Source: CAD feature listing. Evaluate the final solid. Frame: model axes, mm. A direction names the side the tool comes from. Round coordinates to 2 decimals unless told otherwise and drop trailing zeros. Write each loop counter-clockwise with the first axis right and the second up, starting at its lowest first coordinate (ties: lowest second). Pieces come first, ordered by that corner, then holes. Notation, with made-up numbers: M -12,27.5 L 19,27.5 A9 cw 19,35.5 Z; hole C 30.5,0 d3. An arc over 180 degrees is marked long. Answer in a Markdown table with one row per item. Add a question column.
Item 1: Material intervals for probe 1 along Y at (x, z) = (-14.5, 2.85); probe 2 along X at (y, z) = (-22, 0.7); probe 3 along X at (y, z) = (-40, 2.85), sorted ascending.
Item 2: Cut plane C-C on x = 8. Return loops of the section in (y, z), and give its area (3 significant figures).
Item 3: Set-up query: faces 5 (the face through (0, -24, 0)), 6 (the face through (14.222, -27.236, 1.578)). Return all of +Z, -Z, +X, -X, +Y, -Y with unobstructed straight access to the full face (end or side cutting, diameter ignored); none if empty.
Item 4: Mould query, pull axis X, two halves, no side actions, for faces 1 (the face through (0.58, -57.188, 2.465)), 2 (the face through (3, -42, 3.2)), 3 (the face through (11.753, -23.369, 4.087)), 4 (the face through (-15.837, -36.846, 2.465)). Classes: released by +X, released by -X, zero draft, split by the parting line, or undercut.
Item 5: Cut plane D-D on y = -32. Return loops of the section in (x, z).
Item 6: Cut plane B-B on y = -23. Return loops of the section in (x, z).
Item 7: Cut plane A-A on z = 2.3. Return loops of the section in (x, y).
Item 8: Contact query for flat-ended pins moving along their axis: pin 1 (4 mm diameter, centred on x = 12.5, y = -22.5, fed in from +Z); pin 2 (2 mm diameter, centred on x = -12, y = -24, fed in from -Z); pin 3 (2 mm diameter, centred on y = -43, z = 3.5, fed in from -X); pin 4 (5.5 mm diameter, centred on x = -12.29, y = -24.01, fed in from -Z). Output: stop coordinate, or through.
from build123d import *

# Parameters (mm, degrees)
F0_R     = 4
F0_R_2   = 3.25
F0_R_3   = 2.145
F1_DEPTH = 5
F2_DEPTH = 3.2


with BuildPart() as f1:
    # F0 (on Top) → F1 (new body)
    with BuildSketch(Plane.XY):
        with BuildLine():
            ThreePointArc((-10.6575777754, -53.0245751143), (-5.3198116886, -56.1150509582), (0.7539304934, -57.1885702394))
            ThreePointArc((0.7539304934, -57.1885702394), (6.8276726753, -56.1150509582), (12.1654387622, -53.0245751143))
            ThreePointArc((12.1654387622, -53.0245751143), (17.232310235, -37.0535716462), (27.7539304934, -24.013569904))
            ThreePointArc((27.7539304934, -24.013569904), (0.7539304934, -3.2972529395), (-26.2460695066, -24.013569904))
            ThreePointArc((-26.2460695066, -24.013569904), (-15.7244492482, -37.0535716462), (-10.6575777754, -53.0245751143))
        make_face()
        with BuildLine():
            ThreePointArc((4.7539304934, -41.1667175744), (3.5823576181, -43.9951446991), (0.7539304934, -45.1667175744))
            ThreePointArc((0.7539304934, -45.1667175744), (-3.2460695066, -41.1667175744), (0.7539304934, -37.1667175744))
            ThreePointArc((0.7539304934, -37.1667175744), (3.5823576181, -38.3382904496), (4.7539304934, -41.1667175744))
        make_face(mode=Mode.SUBTRACT)
        with Locations((-12.2910695066, -24.013569904)):
            Circle(F0_R, mode=Mode.SUBTRACT)
        with BuildLine():
            ThreePointArc((17.7989304934, -24.013569904), (13.7989304934, -28.013569904), (9.7989304934, -24.013569904))
            ThreePointArc((9.7989304934, -24.013569904), (13.7989304934, -20.013569904), (17.7989304934, -24.013569904))
        make_face(mode=Mode.SUBTRACT)
        with BuildLine():
            ThreePointArc((17.7989304934, -24.013569904), (13.7989304934, -20.013569904), (9.7989304934, -24.013569904))
            ThreePointArc((9.7989304934, -24.013569904), (13.7989304934, -28.013569904), (17.7989304934, -24.013569904))
        make_face()
        with BuildLine():
            ThreePointArc((17.0489304934, -24.013569904), (13.7989304934, -27.263569904), (10.5489304934, -24.013569904))
            ThreePointArc((10.5489304934, -24.013569904), (13.7989304934, -20.763569904), (17.0489304934, -24.013569904))
        make_face(mode=Mode.SUBTRACT)
        with Locations((-12.2910695066, -24.013569904)):
            Circle(F0_R)
        with Locations((-12.2910695066, -24.013569904)):
            Circle(F0_R_2, mode=Mode.SUBTRACT)
        with BuildLine():
            ThreePointArc((17.0489304934, -24.013569904), (13.7989304934, -20.763569904), (10.5489304934, -24.013569904))
            ThreePointArc((10.5489304934, -24.013569904), (13.7989304934, -27.263569904), (17.0489304934, -24.013569904))
        make_face()
        with BuildLine():
            ThreePointArc((15.9439304934, -24.013569904), (13.7989304934, -26.158569904), (11.6539304934, -24.013569904))
            ThreePointArc((11.6539304934, -24.013569904), (13.7989304934, -21.868569904), (15.9439304934, -24.013569904))
        make_face(mode=Mode.SUBTRACT)
        with Locations((-12.2910695066, -24.013569904)):
            Circle(F0_R_2)
        with Locations((-12.2910695066, -24.013569904)):
            Circle(F0_R_3, mode=Mode.SUBTRACT)
        with BuildLine():
            ThreePointArc((0.7539304934, -37.9167175744), (-2.4960695066, -41.1667175744), (0.7539304934, -44.4167175744))
            Line((0.7539304934, -44.4167175744), (0.7539304934, -43.3117175744))
            ThreePointArc((0.7539304934, -43.3117175744), (-1.3910695066, -41.1667175744), (0.7539304934, -39.0217175744))
            Line((0.7539304934, -39.0217175744), (0.7539304934, -37.9167175744))
        make_face()
        with BuildLine():
            Line((0.7539304934, -43.3117175744), (0.7539304934, -44.4167175744))
            ThreePointArc((0.7539304934, -44.4167175744), (3.0520275322, -43.4648146132), (4.0039304934, -41.1667175744))
            ThreePointArc((4.0039304934, -41.1667175744), (3.0520275322, -38.8686205355), (0.7539304934, -37.9167175744))
            Line((0.7539304934, -37.9167175744), (0.7539304934, -39.0217175744))
            ThreePointArc((0.7539304934, -39.0217175744), (2.270674539, -39.6499735287), (2.8989304934, -41.1667175744))
            ThreePointArc((2.8989304934, -41.1667175744), (2.270674539, -42.68346162), (0.7539304934, -43.3117175744))
        make_face()
        with BuildLine():
            ThreePointArc((0.7539304934, -37.1667175744), (-3.2460695066, -41.1667175744), (0.7539304934, -45.1667175744))
            Line((0.7539304934, -45.1667175744), (0.7539304934, -44.4167175744))
            ThreePointArc((0.7539304934, -44.4167175744), (-2.4960695066, -41.1667175744), (0.7539304934, -37.9167175744))
            Line((0.7539304934, -37.9167175744), (0.7539304934, -37.1667175744))
        make_face()
        with BuildLine():
            Line((0.7539304934, -44.4167175744), (0.7539304934, -45.1667175744))
            ThreePointArc((0.7539304934, -45.1667175744), (3.5823576181, -43.9951446991), (4.7539304934, -41.1667175744))
            ThreePointArc((4.7539304934, -41.1667175744), (3.5823576181, -38.3382904496), (0.7539304934, -37.1667175744))
            Line((0.7539304934, -37.1667175744), (0.7539304934, -37.9167175744))
            ThreePointArc((0.7539304934, -37.9167175744), (3.0520275322, -38.8686205355), (4.0039304934, -41.1667175744))
            ThreePointArc((4.0039304934, -41.1667175744), (3.0520275322, -43.4648146132), (0.7539304934, -44.4167175744))
        make_face()
    extrude(amount=F1_DEPTH)

    # F0 (on Top) → F2 (cut)
    with BuildSketch(Plane.XY):
        with BuildLine():
            ThreePointArc((17.0489304934, -24.013569904), (13.7989304934, -20.763569904), (10.5489304934, -24.013569904))
            ThreePointArc((10.5489304934, -24.013569904), (13.7989304934, -27.263569904), (17.0489304934, -24.013569904))
        make_face()
        with BuildLine():
            ThreePointArc((15.9439304934, -24.013569904), (13.7989304934, -26.158569904), (11.6539304934, -24.013569904))
            ThreePointArc((11.6539304934, -24.013569904), (13.7989304934, -21.868569904), (15.9439304934, -24.013569904))
        make_face(mode=Mode.SUBTRACT)
        with Locations((-12.2910695066, -24.013569904)):
            Circle(F0_R_2)
        with Locations((-12.2910695066, -24.013569904)):
            Circle(F0_R_3, mode=Mode.SUBTRACT)
        with BuildLine():
            ThreePointArc((0.7539304934, -37.9167175744), (-2.4960695066, -41.1667175744), (0.7539304934, -44.4167175744))
            Line((0.7539304934, -44.4167175744), (0.7539304934, -43.3117175744))
            ThreePointArc((0.7539304934, -43.3117175744), (-1.3910695066, -41.1667175744), (0.7539304934, -39.0217175744))
            Line((0.7539304934, -39.0217175744), (0.7539304934, -37.9167175744))
        make_face()
        with BuildLine():
            Line((0.7539304934, -43.3117175744), (0.7539304934, -44.4167175744))
            ThreePointArc((0.7539304934, -44.4167175744), (3.0520275322, -43.4648146132), (4.0039304934, -41.1667175744))
            ThreePointArc((4.0039304934, -41.1667175744), (3.0520275322, -38.8686205355), (0.7539304934, -37.9167175744))
            Line((0.7539304934, -37.9167175744), (0.7539304934, -39.0217175744))
            ThreePointArc((0.7539304934, -39.0217175744), (2.270674539, -39.6499735287), (2.8989304934, -41.1667175744))
            ThreePointArc((2.8989304934, -41.1667175744), (2.270674539, -42.68346162), (0.7539304934, -43.3117175744))
        make_face()
    extrude(amount=F2_DEPTH, mode=Mode.SUBTRACT)


solid = f1.part
Results below:
| question | item | result |
|---|---|---|
| 1 | probe 1 | -39.51 to -26.4, -21.63 to -7.83 |
| 1 | probe 2 | -25.62 to -14.84, -9.74 to 11.25, 16.35 to 27.13 |
| 1 | probe 3 | -14.28 to -2.28, 3.79 to 15.78 |
| 2 | outline | M -55.64,0 L -4.25,0 L -4.25,5 L -55.64,5 Z |
| 2 | area | 257 mm2 |
| 3 | face 5 | -Z, +X, -X, +Y, -Y |
| 3 | face 6 | -Z |
| 4 | face 1 | split by the parting line |
| 4 | face 2 | undercut |
| 4 | face 3 | undercut |
| 4 | face 4 | released by -X |
| 5 | outline | M -18.88,0 L 20.39,0 L 20.39,5 L -18.88,5 Z |
| 6 | outline | M -25.95,0 L -15.38,0 L -15.38,3.2 L -14.18,3.2 L -14.18,5 L -25.95,5 Z; M -10.4,3.2 L -9.2,3.2 L -9.2,0 L 10.71,0 L 10.71,3.2 L 11.91,3.2 L 11.91,5 L -10.4,5 Z; M 15.69,3.2 L 16.89,3.2 L 16.89,0 L 27.46,0 L 27.46,5 L 15.69,5 Z |
| 7 | outline | M -26.25,-24.01 A45.34 cw -10.66,-53.02 A17.72 ccw 12.17,-53.02 A45.34 cw 27.75,-24.01 A27.95 ccw Z; hole C -12.29,-24.01 d6.5; hole C 0.75,-41.17 d6.5; hole C 13.8,-24.01 d6.5 |
| 8 | pin 1 | z = 5 |
| 8 | pin 2 | through |
| 8 | pin 3 | x = -13.44 |
| 8 | pin 4 | z = 3.2 |
